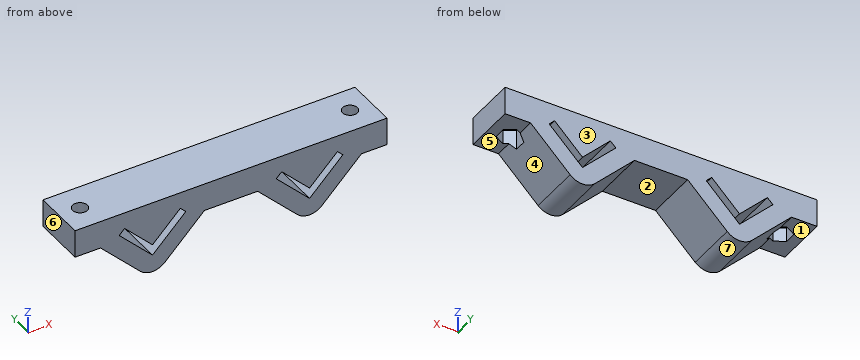
from build123d import *

# Parameters (mm, degrees)
F1_DEPTH = 15
F2_R     = 2.125
F3_DEPTH = 25
F5_DEPTH = 4
F6_R     = 5
F8_DEPTH = 25


with BuildPart() as f1:
    # F0 (on Front) → F1 (new body)
    with BuildSketch(Plane.XZ):
        Polygon((22.182061, 12.7), (15.317939, 12.7), (14.682061, 12.7), (-14.682061, 12.7), (-22.182061, 12.7), (-22.182061, 4.7), (-14.882338, 4.7), (-7.5, -2.682338), (0, -10.182338), (7.5, -2.682338), (14.882338, 4.7), (30.117662, 4.7), (37.5, -2.682338), (45, -10.182338), (52.5, -2.682338), (59.882338, 4.7), (67.182061, 4.7), (67.182061, 12.7), (59.682061, 12.7), (30.317939, 12.7), (29.682061, 12.7), (22.817939, 12.7), align=None)
        Polygon((-9.545942, 6.434672), (-7.990307, 7.990307), (0, 0), (7.990307, 7.990307), (9.545942, 6.434672), (0, -3.11127), align=None, mode=Mode.SUBTRACT)
        Polygon((35.454058, 6.434672), (37.009693, 7.990307), (45, 0), (52.990307, 7.990307), (54.545942, 6.434672), (45, -3.11127), align=None, mode=Mode.SUBTRACT)
    extrude(amount=F1_DEPTH)

    # F2 (on face) → F3 (cut)
    with BuildSketch(Plane.XY.offset(12.7)):
        with Locations((-16.182061, -7.5)):
            Circle(F2_R)
        with Locations((61.182061, -7.5)):
            Circle(F2_R)
    extrude(amount=-F3_DEPTH, mode=Mode.SUBTRACT)

    # F4 (on face) → F5 (cut)
    with BuildSketch(Plane(origin=(0, 0, 4.7), x_dir=(1, 0, 0), z_dir=(0, 0, -1))):
        Polygon((-19.107061, 9.18875), (-19.107061, 5.81125), (-16.182061, 4.122501), (-13.257061, 5.81125), (-13.257061, 9.18875), (-16.182061, 10.877499), align=None)
        Polygon((64.107061, 5.81125), (64.107061, 9.18875), (61.182061, 10.877499), (58.257061, 9.18875), (58.257061, 5.81125), (61.182061, 4.122501), align=None)
    extrude(amount=-F5_DEPTH, mode=Mode.SUBTRACT)

    # F6
    f6_edges = [f1.edges().sort_by_distance(p)[0] for p in [
        (0, -7.5, -10.182338),
        (45, -7.5, -10.182338),
    ]]
    fillet(f6_edges, radius=F6_R)

    # F7 (on face) → F8 (cut)
    with BuildSketch(Plane(origin=(0, 0, 8.7), x_dir=(1, 0, 0), z_dir=(0, 0, -1))):
        Polygon((-19.107061, 9.18875), (-19.107061, 5.81125), (-16.182061, 4.122501), (-13.257061, 5.81125), (-13.257061, 9.18875), (-16.182061, 10.877499), align=None)
        Polygon((64.107061, 5.81125), (64.107061, 9.18875), (61.182061, 10.877499), (58.257061, 9.18875), (58.257061, 5.81125), (61.182061, 4.122501), align=None)
    extrude(amount=F8_DEPTH, mode=Mode.SUBTRACT)


solid = f1.part
Here's how the part is built. I have some questions about the finished solid (model axes, mm). Face numbers are marked on the shaded views. A direction names the side the tool comes from. Round coordinates to 2 decimals unless told otherwise and drop trailing zeros. Loops run counter-clockwise (first coordinate to the right, second up) from the corner with the lowest first, then second, coordinate; pieces in that order, holes last. Notation, with made-up numbers: (75.25, -8) - (104.25, -8) arc R29 cw to (104.25, 30) - close; hole circle Ø6 at (61, 77.25). An arc over 180 degrees is marked (long way). One line per question, with ' | ' between items. Start each with the question number.
Q1. I want a section at B-B (z = -4). Write out the boundary of the cut face in (x, y).
Q2. I want a section at D-D (z = 9.75). Write out the boundary of the cut face in (x, y) (3 decimals), then the cut area to 3 significant figures.
Q3. I want a section at C-C (y = -7.5). State how many separate pieces and enclosed holes the cut face has, then the cut area to 3 significant figures.
Q4. For the marked faces 1, 2 and 3, which set-ups out of +Z, -Z, +X, -X, +Y, -Y let a thin tool reach every point of the face, with its end or its side?
Q5. We'd pull the mould along X, two halves only. Please class the marked faces 4, 5, 6 and 7: +X half, -X half, draft (parallel to the pull), parting line (faces both ways), or undercut.
Q6. Will these pins go through, and if not, where does the flat tip stop? pin 1 (2 mm diameter, centred on y = -5, z = -4.5, fed in from -X); pin 2 (3 mm diameter, centred on y = -11.5, z = -4.5, fed in from +X); pin 3 (6 mm diameter, centred on x = -20, y = -10, fed in from -Z).
Q7. Please list where these lines run through material, in increasing order: line 1 (X direction, y = -14, z = 2.5); line 2 (Z direction, x = -17, y = -3.25); line 3 (X direction, y = -7, z = -3). Write a range as [from, to].
Q8. I want a section at A-A (y = -13). Write out the boundary of the cut face in (x, z), then the cut area to 3 significant figures.
Response values:
1) outline: (-6.18, -15) - (6.18, -15) - (6.18, 0) - (-6.18, 0) - close; (38.82, -15) - (51.18, -15) - (51.18, 0) - (38.82, 0) - close
2) outline: (-22.182, -15) - (67.182, -15) - (67.182, 0) - (-22.182, 0) - close; hole circle Ø4.25 at (-16.182, -7.5); hole circle Ø4.25 at (61.182, -7.5) | area: 1,310 mm²
3) separate pieces: 3 | enclosed holes: 2 | area: 955 mm²
4) face 1: -Z, -X, +Y, -Y | face 2: -Z, +Y, -Y | face 3: +Z, -Z, +X, -X, +Y
5) face 4: +X half | face 5: draft | face 6: -X half | face 7: undercut
6) pin 1: stops at x = -6.68 | pin 2: stops at x = 52.18 | pin 3: stops at z = 4.7
7) line 1: x = [-12.68, -5.61], [-2.5, 2.5], [5.61, 12.68], [32.32, 39.39], [42.5, 47.5], [50.61, 57.68] | line 2: z = [4.7, 12.7] | line 3: x = [-7.18, -0.11], [0.11, 7.18], [37.82, 44.89], [45.11, 52.18]
8) outline: (-22.18, 4.7) - (-14.88, 4.7) - (-3.54, -6.65) arc R5 ccw to (3.54, -6.65) - (14.88, 4.7) - (30.12, 4.7) - (41.46, -6.65) arc R5 ccw to (48.54, -6.65) - (59.88, 4.7) - (67.18, 4.7) - (67.18, 12.7) - (-22.18, 12.7) - close; hole (-9.55, 6.43) - (0, -3.11) - (9.55, 6.43) - (7.99, 7.99) - (0, 0) - (-7.99, 7.99) - close; hole (35.45, 6.43) - (45, -3.11) - (54.55, 6.43) - (52.99, 7.99) - (45, 0) - (37.01, 7.99) - close | area: 1,040 mm²
